Source: CAD feature listing. Evaluate the final solid. Frame: model axes, mm. Face numbers are marked on the shaded views. A direction names the side the tool comes from. Give positions to 0.01 mm unless a question says otherwise; leave off trailing zeros. Loops run counter-clockwise (first coordinate to the right, second up) from the corner with the lowest first, then second, coordinate; pieces in that order, holes last. Notation, with made-up numbers: (-15.75, 48) -> (-1.75, 48) arc R20 ccw to (-1.75, 82) -> close; hole circle Ø6 at (-26, 34). An arc over 180 degrees is marked (long way). Put each result on its own line as item: value.
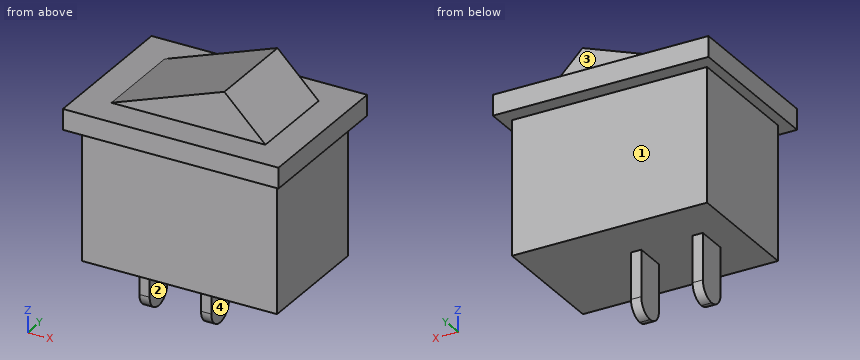
Autodesk Inventor part; units mm, degrees
ref_plane "YZ Plane" through (0, 0, 0) normal (1, 0, 0) x (0, 1, 0)
ref_plane "XZ Plane" through (0, 0, 0) normal (0, 1, 0) x (-1, 0, 0)
ref_plane "XY Plane" through (0, 0, 0) normal (0, 0, 1) x (1, 0, 0)
sketch "スケッチ1" plane through (0, 0, 0) normal (0, 0, 1) x (1, 0, 0)
  line L0 (-9.1992, 6.0057) -> (9.8008, 6.0057)
  line L1 (9.8008, 6.0057) -> (9.8008, -5.9943)
  line L2 (9.8008, -5.9943) -> (-9.1992, -5.9943)
  line L3 (-9.1992, -5.9943) -> (-9.1992, 6.0057)
  dimension "d0" = 19
  dimension "d1" = 12
extrude "押し出し1" add sketch "スケッチ1" along normal blind 13
sketch "スケッチ2" plane through (0, 0, 13) normal (0, 0, 1) x (1, 0, 0)
  line L0 (-9.1992, 6.0057) -> (9.8008, 6.0057)
  line L1 (-9.1992, -5.9943) -> (-9.1992, 6.0057)
  line L2 (-10.1992, 7.5057) -> (10.8008, 7.5057)
  line L3 (10.8008, 7.5057) -> (10.8008, -7.4943)
  line L4 (10.8008, -7.4943) -> (-10.1992, -7.4943)
  line L5 (-10.1992, -7.4943) -> (-10.1992, 7.5057)
  dimension "d4" = 21
  dimension "d5" = 15
  dimension "d6" = 1.5
  dimension "d7" = 1
extrude "押し出し2" add sketch "スケッチ2" along normal blind 2
sketch "スケッチ3" plane through (0, 0, 15) normal (0, 0, 1) x (1, 0, 0)
  line L0 (-10.1992, 7.5057) -> (10.8008, 7.5057)
  line L1 (-10.1992, -7.4943) -> (-10.1992, 7.5057)
  line L2 (-7.1992, 4.5057) -> (7.8008, 4.5057)
  line L3 (7.8008, 4.5057) -> (7.8008, -4.4943)
  line L4 (7.8008, -4.4943) -> (-7.1992, -4.4943)
  line L5 (-7.1992, -4.4943) -> (-7.1992, 4.5057)
  dimension "d10" = 9
  dimension "d11" = 15
  dimension "d12" = 3
  dimension "d13" = 3
extrude "押し出し3" add sketch "スケッチ3" along normal blind 4
chamfer "面取り1" distance 4 distance2 11 1 edges at (-7.1992, 0.0057, 19) measured on face at (-7.1992, -1.4943, 16.3333)
chamfer "面取り2" distance 4 distance2 4 1 edges at (7.8008, 0.0057, 19) measured on face at (7.8008, 1.5057, 16.3333)
sketch "スケッチ4" plane through (0, 0, 0) normal (0, 0, -1) x (-1, 0, 0)
  line L0 (9.1992, 6.0057) -> (-9.8008, 6.0057)
  line L1 (9.1992, -5.9943) -> (9.1992, 6.0057)
  line L2 (-0.8008, 1.5057) -> (0.1992, 1.5057)
  line L3 (0.1992, 1.5057) -> (0.1992, -1.4943)
  line L4 (0.1992, -1.4943) -> (-0.8008, -1.4943)
  line L5 (-0.8008, -1.4943) -> (-0.8008, 1.5057)
  line L6 (5.1992, 1.5057) -> (6.1992, 1.5057)
  line L7 (6.1992, 1.5057) -> (6.1992, -1.4943)
  line L8 (6.1992, -1.4943) -> (5.1992, -1.4943)
  line L9 (5.1992, -1.4943) -> (5.1992, 1.5057)
  dimension "d20" = 9
  dimension "d21" = 1
  dimension "d22" = 3
  dimension "d23" = 4.5
  dimension "d24" = 1
  dimension "d25" = 5
extrude "押し出し4" add sketch "スケッチ4" along normal blind 6
fillet "フィレット1" radius 1.5 4 edges at (0.3008, 1.5057, -6) (0.3008, -1.4943, -6) (-5.6992, -1.4943, -6) (-5.6992, 1.5057, -6)
properties part number "sw" material "ABS Plastic"
(1) Section B-B on x = 6.5. Return loops of the section in (y, z).
Calculated:
outline: (-7.49, 13) -> (-5.99, 13) -> (-5.99, 0) -> (6.01, 0) -> (6.01, 13) -> (7.51, 13) -> (7.51, 15) -> (4.51, 15) -> (4.51, 16.3) -> (-4.49, 16.3) -> (-4.49, 15) -> (-7.49, 15) -> close
(2) Section A-A on y = -5.5. Return loops of the section in (x, z), then the cut area to 3 significant figures.
Calculated:
outline: (-10.2, 13) -> (-9.2, 13) -> (-9.2, 0) -> (9.8, 0) -> (9.8, 13) -> (10.8, 13) -> (10.8, 15) -> (-10.2, 15) -> close
area: 289 mm²
(3) Line query: probe 1 along X at (y, z) = (0.75, -4.5); probe 2 along Z at (x, y) = (1.25, -4.75); probe 3 along X at (y, z) = (-1.5, 7.5). Output: solid intervals per line, ascending. Write a range as from..to.
Calculated:
probe 1: x = -6.2..-5.2, -0.2..0.8
probe 2: z = 0..15
probe 3: x = -9.2..9.8
(4) Section C-C on z = 4.25. Return loops of the section in (x, y), then the cut area to 3 significant figures.
Calculated:
outline: (-9.2, -5.99) -> (9.8, -5.99) -> (9.8, 6.01) -> (-9.2, 6.01) -> close
area: 228 mm²
(5) First-contact query: P1, Ø2.5, axis at y = -0.5, z = -3, coming from the +X side; P2, Ø4.5, axis at x = 2.5, z = 17.5, coming from the +Y side; P3, Ø2.5, axis at y = -0.5, z = -3.5, coming from the -X side. Flat tips, straight axial feed; report the tip coordinate or a pass-through.
Calculated:
P1: stops at x = 0.8
P2: stops at y = 4.51
P3: stops at x = -6.2
(6) Reachability of the marked faces 1, 2, 3 and 4 from +Z, -Z, +X, -X, +Y, -Y: full face, straight path, thin tool, end or side. Return the list, or none.
Calculated:
face 1: -Z, +X, -X, +Y
face 2: -Z, +Y, -Y
face 3: +Z, +X, -X, +Y
face 4: -Z, +X, +Y, -Y
